Check sheet for the drawn part. Datum: minimum x, y, z corner. Units: mm. A direction names the side the tool comes from. Round coordinates to 2 decimals unless told otherwise and drop trailing zeros. Loops run counter-clockwise (first coordinate to the right, second up) from the corner with the lowest first, then second, coordinate; pieces in that order, holes last.
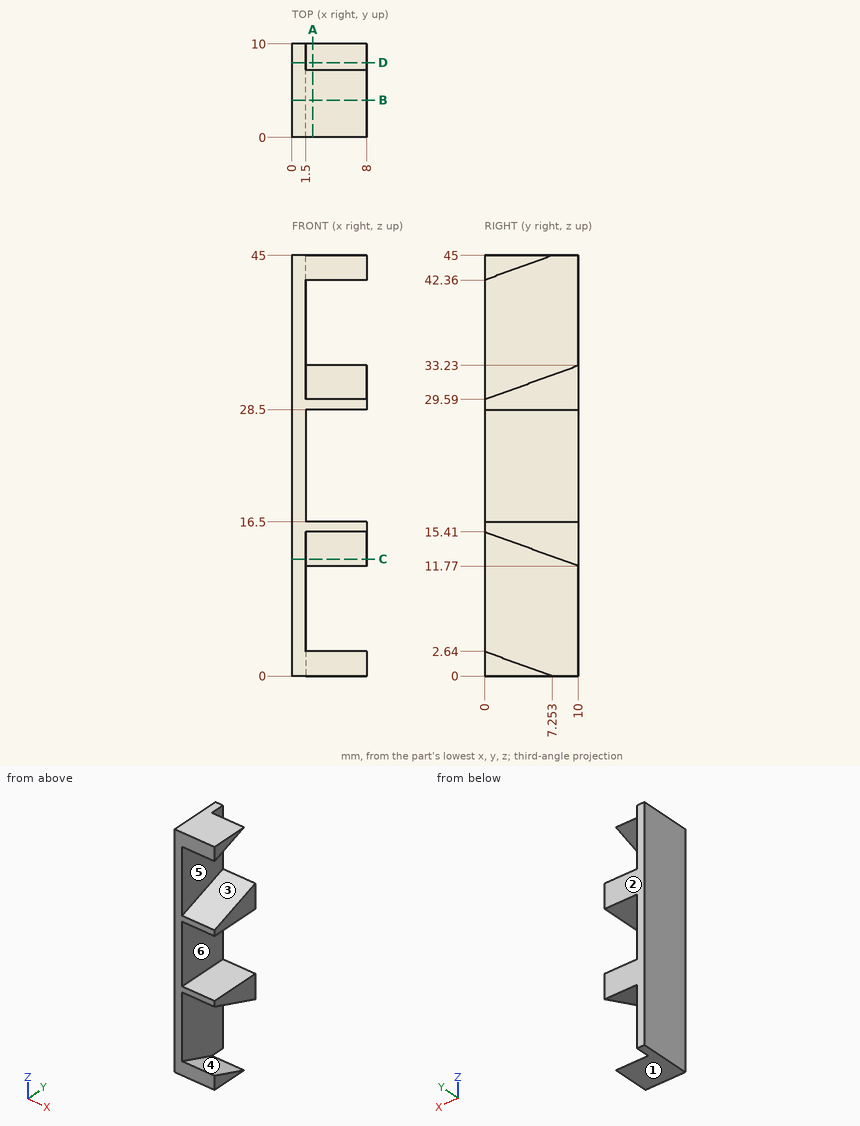
1) Gauge pin test, flat end, axial feed: pin 1 (6 mm diameter, centred on y = 5.5, z = 6.5, fed in from +X). Record the tip position at first contact, or that the pin passes through.
Report:
pin 1: stops at x = 1.5
2) Sectioned sample at A-A, the plane x = 2.25. Record the cut outline in (y, z).
Report:
outline: (0, 0) - (7.25, 0) - (0, 2.64) - close; (0, 15.41) - (10, 11.77) - (10, 16.5) - (0, 16.5) - close; (0, 28.5) - (10, 28.5) - (10, 33.23) - (0, 29.59) - close; (0, 42.36) - (7.25, 45) - (0, 45) - close
3) Access from +Z, -Z, +X, -X, +Y, -Y to the whole of each face (thin tool, end or side, straight path). Record for the marked faces 4, 5 and 6.
Report:
face 4: +X, +Y
face 5: +X
face 6: +X, +Y, -Y
4) Scan lines: line 1 along Z through (x, y) = (4.25, 2.5); line 2 along Z through (x, y) = (4.5, 4.5); line 3 along X through (y, z) = (6, 6.5). Record each from-to range of solid material in increasing order.
Report:
line 1: z = 0 to 1.73, 14.5 to 16.5, 28.5 to 30.5, 43.27 to 45
line 2: z = 0 to 1, 13.77 to 16.5, 28.5 to 31.23, 44 to 45
line 3: x = 0 to 1.5
5) Sectioned sample at B-B, the plane y = 4. Record the cut outline in (x, z), then the cut area to 3 significant figures.
Report:
outline: (0, 0) - (8, 0) - (8, 1.18) - (1.5, 1.18) - (1.5, 13.95) - (8, 13.95) - (8, 16.5) - (1.5, 16.5) - (1.5, 28.5) - (8, 28.5) - (8, 31.05) - (1.5, 31.05) - (1.5, 43.82) - (8, 43.82) - (8, 45) - (0, 45) - close
area: 116 mm2
6) Sectioned sample at D-D, the plane y = 8. Record the cut outline in (x, z).
Report:
outline: (0, 0) - (1.5, 0) - (1.5, 12.5) - (8, 12.5) - (8, 16.5) - (1.5, 16.5) - (1.5, 28.5) - (8, 28.5) - (8, 32.5) - (1.5, 32.5) - (1.5, 45) - (0, 45) - close
7) Mould release check, pull along Z, two halves, no side actions. Record for the marked faces 1, 2 and 3: +Z half, -Z half, draft (parallel to the pull), parting line (faces both ways), or undercut.
Report:
face 1: -Z half
face 2: draft
face 3: undercut
8) Sectioned sample at C-C, the plane z = 12.5. Record the cut outline in (x, y) (1 decimal).
Report:
outline: (0, 0) - (1.5, 0) - (1.5, 8) - (8, 8) - (8, 10) - (0, 10) - close
